```python
from build123d import *

# Parameters (mm, degrees)
SKETCH_1_R      = 2
SKETCH_1_R_2    = 2.08
SKETCH_1_R_3    = 8.75
SKETCH_1_R_4    = 4.5
EXTRUDE_2_DEPTH = 2


with BuildPart() as part:
    # 草图1 → 凸台-拉伸2 (new body)
    with BuildSketch(Plane.XY):
        with BuildLine():
            Line((41.5, 13.75), (41.5, 17))
            Line((41.5, 17), (37, 17))
            Line((37, 17), (37, 19))
            Line((37, 19), (30, 19))
            Line((30, 19), (30, 17))
            Line((30, 17), (25.488968202, 17))
            ThreePointArc((25.488968202, 17), (0, 27.55787632), (-25.488968202, 17))
            Line((-25.488968202, 17), (-30, 17))
            Line((-30, 17), (-30, 19))
            Line((-30, 19), (-37, 19))
            Line((-37, 19), (-37, 17))
            Line((-37, 17), (-41.5, 17))
            Line((-41.5, 17), (-41.5, 13.75))
            Line((-41.5, 13.75), (-43.5, 13.75))
            Line((-43.5, 13.75), (-43.5, 8.75))
            Line((-43.5, 8.75), (-41.5, 8.75))
            Line((-41.5, 8.75), (-41.5, 1.5))
            Line((-41.5, 1.5), (-39, 1.5))
            Line((-39, 1.5), (-39, 3))
            Line((-39, 3), (-36.4, 3))
            Line((-36.4, 3), (-36.4, 1.5))
            Line((-36.4, 1.5), (-33.4, 1.5))
            Line((-33.4, 1.5), (-33.4, -1.5))
            Line((-33.4, -1.5), (-36.4, -1.5))
            Line((-36.4, -1.5), (-36.4, -3))
            Line((-36.4, -3), (-39, -3))
            Line((-39, -3), (-39, -1.5))
            Line((-39, -1.5), (-41.5, -1.5))
            Line((-41.5, -1.5), (-41.5, -8.75))
            Line((-41.5, -8.75), (-43.5, -8.75))
            Line((-43.5, -8.75), (-43.5, -13.75))
            Line((-43.5, -13.75), (-41.5, -13.75))
            Line((-41.5, -13.75), (-41.5, -17))
            Line((-41.5, -17), (-41.5, -48.49787632))
            Line((-41.5, -48.49787632), (-39, -48.49787632))
            Line((-39, -48.49787632), (-39, -46.99787632))
            Line((-39, -46.99787632), (-36.4, -46.99787632))
            Line((-36.4, -46.99787632), (-36.4, -48.49787632))
            Line((-36.4, -48.49787632), (-33.4, -48.49787632))
            Line((-33.4, -48.49787632), (-33.4, -51.49787632))
            Line((-33.4, -51.49787632), (-36.4, -51.49787632))
            Line((-36.4, -51.49787632), (-36.4, -52.99787632))
            Line((-36.4, -52.99787632), (-39, -52.99787632))
            Line((-39, -52.99787632), (-39, -51.49787632))
            Line((-39, -51.49787632), (-41.5, -51.49787632))
            Line((-41.5, -51.49787632), (-41.5, -58.74787632))
            Line((-41.5, -58.74787632), (-43.5, -58.74787632))
            Line((-43.5, -58.74787632), (-43.5, -63.74787632))
            Line((-43.5, -63.74787632), (-41.5, -63.74787632))
            Line((-41.5, -63.74787632), (-41.5, -69.55787632))
            Line((-41.5, -69.55787632), (-35, -69.55787632))
            ThreePointArc((-35, -69.55787632), (-32.878679656, -70.436555977), (-32, -72.55787632))
            Line((-32, -72.55787632), (-32, -74.55787632))
            ThreePointArc((-32, -74.55787632), (-25, -81.55787632), (-18, -74.55787632))
            Line((-18, -74.55787632), (25.488968202, -17))
            Line((25.488968202, -17), (30, -17))
            Line((30, -17), (30, -19))
            Line((30, -19), (37, -19))
            Line((37, -19), (37, -17))
            Line((37, -17), (41.5, -17))
            Line((41.5, -17), (41.5, -13.75))
            Line((41.5, -13.75), (43.5, -13.75))
            Line((43.5, -13.75), (43.5, -8.75))
            Line((43.5, -8.75), (41.5, -8.75))
            Line((41.5, -8.75), (41.5, -1.5))
            Line((41.5, -1.5), (39, -1.5))
            Line((39, -1.5), (39, -3))
            Line((39, -3), (36.4, -3))
            Line((36.4, -3), (36.4, -1.5))
            Line((36.4, -1.5), (33.4, -1.5))
            Line((33.4, -1.5), (33.4, 1.5))
            Line((33.4, 1.5), (36.4, 1.5))
            Line((36.4, 1.5), (36.4, 3))
            Line((36.4, 3), (39, 3))
            Line((39, 3), (39, 1.5))
            Line((39, 1.5), (41.5, 1.5))
            Line((41.5, 1.5), (41.5, 8.75))
            Line((41.5, 8.75), (43.5, 8.75))
            Line((43.5, 8.75), (43.5, 13.75))
            Line((43.5, 13.75), (41.5, 13.75))
        make_face()
        with Locations((0, -15)):
            Circle(SKETCH_1_R, mode=Mode.SUBTRACT)
        with Locations((-12.990381057, -7.5)):
            Circle(SKETCH_1_R, mode=Mode.SUBTRACT)
        with Locations((-12.990381057, 7.5)):
            Circle(SKETCH_1_R, mode=Mode.SUBTRACT)
        with Locations((0, 15)):
            Circle(SKETCH_1_R, mode=Mode.SUBTRACT)
        with Locations((12.990381057, 7.5)):
            Circle(SKETCH_1_R, mode=Mode.SUBTRACT)
        with Locations((12.990381057, -7.5)):
            Circle(SKETCH_1_R, mode=Mode.SUBTRACT)
        with Locations((-13.53, 0)):
            Circle(SKETCH_1_R_2, mode=Mode.SUBTRACT)
        with Locations((6.765, 11.717323713)):
            Circle(SKETCH_1_R_2, mode=Mode.SUBTRACT)
        with Locations((6.765, -11.717323713)):
            Circle(SKETCH_1_R_2, mode=Mode.SUBTRACT)
        Circle(SKETCH_1_R_3, mode=Mode.SUBTRACT)
        with Locations((-25, -74.55787632)):
            Circle(SKETCH_1_R_4, mode=Mode.SUBTRACT)
    extrude(amount=EXTRUDE_2_DEPTH)


solid = part.part
```
For this review, take the finished solid that the model builds, in its own axes (mm). Give positions to 0.01 mm unless a question says otherwise; leave off trailing zeros. Write each loop counter-clockwise with the first axis right and the second up, starting at its lowest first coordinate (ties: lowest second). Pieces come first, ordered by that corner, then holes. Notation, with made-up numbers: M 62,-26.75 L 89,-26.75 A16 cw 89,-3.75 Z; hole C 40,18 d8. An arc over 180 degrees is marked long. Answer as CSV lines item,"result".
1. Consider section A-A, the plane y = 15. Write out the cut boundary in (x, z), then the cut area to 3 significant figures.
Findings:
outline,"M -41.5,0 L -2,0 L -2,2 L -41.5,2 Z; M 2,0 L 41.5,0 L 41.5,2 L 2,2 Z"
area,"158 mm2"
2. Consider section C-C, the plane x = 0. Write out the cut boundary in (y, z).
Findings:
outline,"M -50.73,0 L -17,0 L -17,2 L -50.73,2 Z; M -13,0 L -8.75,0 L -8.75,2 L -13,2 Z; M 8.75,0 L 13,0 L 13,2 L 8.75,2 Z; M 17,0 L 27.56,0 L 27.56,2 L 17,2 Z"
3. Draft analysis for pull direction X (two halves, no side actions). For faces 1 (the cylindrical face through (-25.154, -81.556, 0.986)), 2 (the cylindrical face through (12.73, 9.483, 0.986)), 3 (the cylindrical face through (-6.944, -5.324, 0.986)), 4 (the flat face through (-10, -14, 0)), state which applies: +X half, -X half, draft (parallel to the pull), parting line (faces both ways), or undercut.
Findings:
face 1,"parting line"
face 2,"undercut"
face 3,"undercut"
face 4,"draft"
4. Consider section D-D, the plane z = 1.6. Count the separate pieces of the cut face and the enclosed holes in it, then the cut area to 3 significant figures.
Findings:
separate pieces,"1"
enclosed holes,"11"
area,"5,400 mm2"
5. Wall thickness on line 1 (X direction, y = -8, z = 0.6); line 2 (Y direction, x = 6.5, z = 1); line 3 (Y direction, x = 13, z = 0.25): over which ranges is each line inside the solid? List them lowest first.
Findings:
line 1,"x = -41.5 to -14.93, -11.05 to -3.54, 3.54 to 11.05, 14.93 to 41.5"
line 2,"y = -42.13 to -13.78, -9.65 to -5.86, 5.86 to 9.65, 13.78 to 26.97"
line 3,"y = -33.53 to -9.5, -5.5 to 5.5, 9.5 to 25.13"
6. For pin 1 (0.6 mm diameter, centred on y = -56, z = 0.5, fed in from -X); pin 2 (1 mm diameter, centred on y = -0.5, z = 1, fed in from -X); pin 3 (1 mm diameter, centred on x = -28, z = 1.5, fed in from +Y), all flat-tipped, find the tip position at first contact; note any pin that passes through.
Findings:
pin 1,"stops at x = -41.5"
pin 2,"stops at x = -33.4"
pin 3,"stops at y = 17"
7. Consider section B-B, the plane y = 0. Write out the cut boundary in (x, z), then the cut area to 3 significant figures.
Findings:
outline,"M -33.4,0 L -15.61,0 L -15.61,2 L -33.4,2 Z; M -11.45,0 L -8.75,0 L -8.75,2 L -11.45,2 Z; M 8.75,0 L 33.4,0 L 33.4,2 L 8.75,2 Z"
area,"90.3 mm2"
